The listing builds one solid part. Answer for the finished solid, in the listing's coordinates (mm). Face numbers are marked on the shaded views. A direction names the side the tool comes from. Coordinates: 2 decimals unless noted, no trailing zeros. Order: outer loops, then holes, each group sorted by start corner. A loop starts at its lowest first (then second) coordinate and runs counter-clockwise, first axis right, second up. Notation, with made-up numbers: M 54,61 L 60,61 A20 cw 60,88 Z; hole C 54,85 d1. An arc over 180 degrees is marked long. One line per item, written item: value. Start each with the question number.
Q1. For the marked faces 4, 5 and 6, determine the directions among +Z, -Z, +X, -X, +Y, -Y from which every point of the face is accessible in a straight line to the end or side of a thin tool.
Q2. The part is cut by section C-C on z = 22. Give the vertices of the cut face in (x, y), then the cut area to 3 significant figures.
Q3. The part is cut by section B-B on x = 0. Give the vertices of the cut face in (y, z), then the cut area to 3 significant figures.
Q4. The part is cut by section A-A on z = 2.5. Give the vertices of the cut face in (x, y).
Q5. Straight lines are drawn through the part: line 1 along X through (y, z) = (1, 2); line 2 along X through (y, z) = (8, 4); line 3 along Y through (x, z) = (0, 27). For each, find the intervals that lie inside material, in ascending order. Write a range as [from, to].
Q6. Determine the mould class of the marked faces 1, 2 and 3 for opening direction Y: pulls with the +Y half, pulls with the -Y half, needs draft (parallel to the pull), parting line crosses it, or undercut.
Q7. Each of these flat-tipped pins is pushed along its axis until it touches: pin 1 Ø8 at (x, y) = (0, 0) entering from +Z; pin 2 Ø10 at (x, y) = (-23.5, 3) entering from -Z; pin 3 Ø1 at (x, y) = (0.5, -10) entering from -Z. Where does it stop, or does it pass through?
Q8. The part is cut by section D-D on y = 0. Give the vertices of the cut face in (x, z), then the cut area to 3 significant figures.
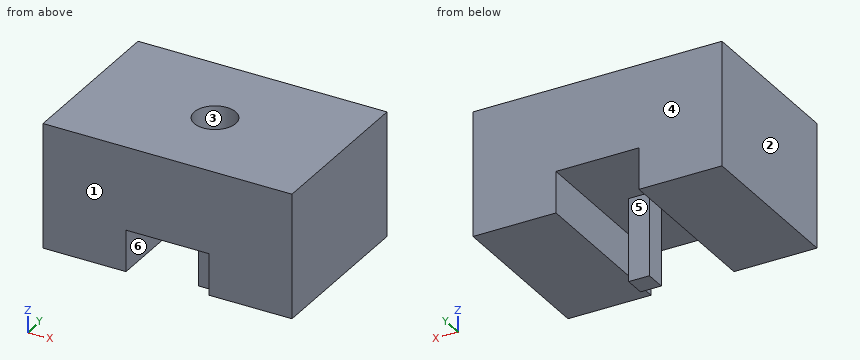
Autodesk Inventor part; units mm, degrees
ref_plane "YZ Plane" through (0, 0, 0) normal (1, 0, 0) x (0, 1, 0)
ref_plane "XZ Plane" through (0, 0, 0) normal (0, 1, 0) x (-1, 0, 0)
ref_plane "XY Plane" through (0, 0, 0) normal (0, 0, 1) x (1, 0, 0)
sketch "Sketch1" plane through (0, 0, 0) normal (0, 0, 1) x (1, 0, 0)
  line L0 (-30, 20) -> (30, 20)
  line L1 (30, 20) -> (30, -20)
  line L2 (30, -20) -> (-30, -20)
  line L3 (-30, -20) -> (-30, 20)
  point P0 (0, 0)
  dimension "d0" = 60
  dimension "d1" = 30
  dimension "d2" = 40
  dimension "d3" = 20
extrude "Extrusion1" add sketch "Sketch1" along normal blind 30
sketch "Sketch3" plane through (-30, 20, 0) normal (0, 1, 0) x (1, 0, 0)
  line L0 (0, 0) -> (60, 0)
  line L1 (20, 0) -> (20, -10)
  line L2 (20, -10) -> (40, -10)
  line L3 (40, -10) -> (40, 0)
  line L4 (20, 0) -> (40, 0)
  point P0 (30, 0)
  point P1 (30, 0)
  dimension "d9" = 20
  dimension "d10" = 10
  dimension "d11" = 10
extrude "Extrusion3" cut sketch "Sketch3" against normal through all
sketch "Sketch5" plane through (10, 20, 10) normal (0, 0, -1) x (-1, 0, 0)
  line L0 (12.5, -22.5) -> (7.5, -22.5)
  line L1 (7.5, -22.5) -> (7.5, -17.5)
  line L2 (7.5, -17.5) -> (12.5, -17.5)
  line L3 (12.5, -17.5) -> (12.5, -22.5)
  point P0 (10, -20)
  point P1 (7.5, -20)
  dimension "d17" = 2.5
  dimension "d18" = 5
  dimension "d19" = 5
  dimension "d20" = 2.5
extrude "Extrusion5" add sketch "Sketch5" along normal blind 20
sketch "Sketch6" plane through (0, 0, 30) normal (0, 0, 1) x (1, 0, 0)
  circle A0 centre (0, 0) radius 5
  dimension "d23" = 10
extrude "Extrusion6" cut sketch "Sketch6" against normal blind 10
properties part number "trzymaczka"
Output:
1. face 4: +Z, -Z, +X, -X, +Y
1. face 5: -Z, +Y
1. face 6: -Z, +Y, -Y
2. outline: M -30,-20 L 30,-20 L 30,20 L -30,20 Z; hole C 0,0 d10
2. area: 2,320 mm^2
3. outline: M -20,10 L -2.5,10 L -2.5,-10 L 2.5,-10 L 2.5,10 L 20,10 L 20,30 L 5,30 L 5,20 L -5,20 L -5,30 L -20,30 Z
3. area: 800 mm^2
4. outline: M -30,-20 L -10,-20 L -10,20 L -30,20 Z; M -2.5,-2.5 L 2.5,-2.5 L 2.5,2.5 L -2.5,2.5 Z; M 10,-20 L 30,-20 L 30,20 L 10,20 Z
5. line 1: x = [-30, -10], [-2.5, 2.5], [10, 30]
5. line 2: x = [-30, -10], [10, 30]
5. line 3: y = [-20, -5], [5, 20]
6. face 1: pulls with the -Y half
6. face 2: needs draft
6. face 3: undercut
7. pin 1: stops at z = 20
7. pin 2: stops at z = 0
7. pin 3: stops at z = 10
8. outline: M -30,0 L -10,0 L -10,10 L -2.5,10 L -2.5,-10 L 2.5,-10 L 2.5,10 L 10,10 L 10,0 L 30,0 L 30,30 L 5,30 L 5,20 L -5,20 L -5,30 L -30,30 Z
8. area: 1,600 mm^2
